Job drawing, mm, ordinate dimensions from the low corner. One solid piece. Round coordinates to 2 decimals unless told otherwise and drop trailing zeros. Write each loop counter-clockwise with the first axis right and the second up, starting at its lowest first coordinate (ties: lowest second). Pieces come first, ordered by that corner, then holes.
1) Saw through at B-B on z = 101.5. Write the cut outline in (x, y) (3 decimals).
2) Saw through at C-C on y = 1.1. Write the cut outline in (x, z), and give its area (3 significant figures).
3) Saw through at A-A on x = 166. Write the cut outline in (y, z) (3 decimals), and give its area (3 significant figures).
4) Flat gauge pin, fed straight in: pin 1 (1 mm diameter, centred on x = 126.5, y = 1.5, fed in from -Z). Where does the tip first touch, or does it go through?
5) Drill centre lines: L1, parallel to X at y = 0.6, z = 109.5; L2, parallel to Z at x = 218.5, y = 3; L3, parallel to X at y = 2.95, z = 51. Where is each one in solid material? Low to high.
6) Pull direction Y, two halves, no side cores. Call the marked faces 1 and 2: +Y half, -Y half, draft (parallel to the pull), parting line (faces both ways), or undercut.
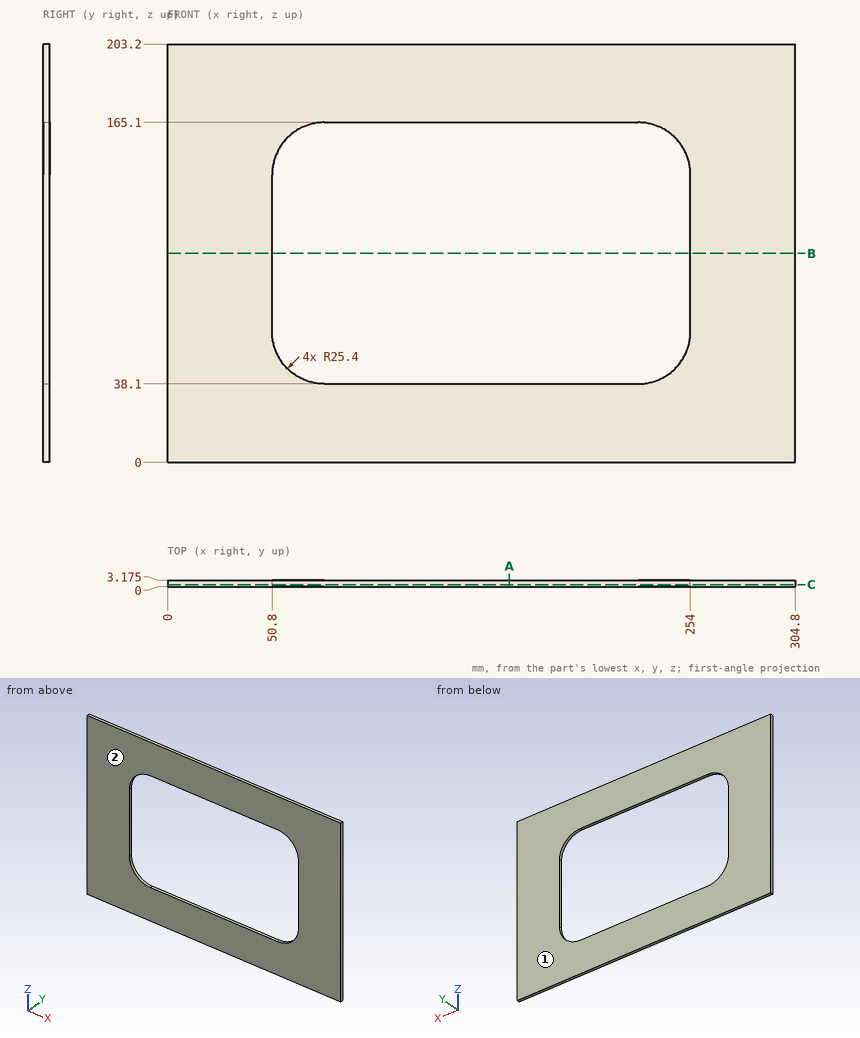
Completed:
1. outline: (0, 0) - (50.8, 0) - (50.8, 3.175) - (0, 3.175) - close; (254, 0) - (304.8, 0) - (304.8, 3.175) - (254, 3.175) - close
2. outline: (0, 0) - (304.8, 0) - (304.8, 203.2) - (0, 203.2) - close; hole (50.8, 63.5) arc R25.4 ccw to (76.2, 38.1) - (228.6, 38.1) arc R25.4 ccw to (254, 63.5) - (254, 139.7) arc R25.4 ccw to (228.6, 165.1) - (76.2, 165.1) arc R25.4 ccw to (50.8, 139.7) - close
2. area: 36,700 mm2
3. outline: (0, 0) - (3.175, 0) - (3.175, 38.1) - (0, 38.1) - close; (0, 165.1) - (3.175, 165.1) - (3.175, 203.2) - (0, 203.2) - close
3. area: 242 mm2
4. pin 1: stops at z = 0
5. L1: x = 0 to 50.8, 254 to 304.8
5. L2: z = 0 to 38.1, 165.1 to 203.2
5. L3: x = 0 to 54.09, 250.71 to 304.8
6. face 1: +Y half
6. face 2: -Y half
